CAD build for the part. Positions are in the model's coordinates, mm. A direction names the side the tool comes from. Round coordinates to 2 decimals unless told otherwise and drop trailing zeros. Write each loop counter-clockwise with the first axis right and the second up, starting at its lowest first coordinate (ties: lowest second). Pieces come first, ordered by that corner, then holes. Notation, with made-up numbers: (-4.5, -24.75) -> (15.5, -24.75) arc R19 cw to (15.5, 3.25) -> close; hole circle Ø10 at (-15, 42). An arc over 180 degrees is marked (long way). Answer in a Markdown table with one row per item. Add a question column.
```python
from build123d import *

# Parameters (mm, degrees)
SKETCH1_W                 = 79
SKETCH1_H                 = 62
SKETCH1_W_2               = 69
SKETCH1_H_2               = 52
BOSS_EXTRUDE1_DEPTH       = 24.3
BOSS_EXTRUDE2_START       = -5
BOSS_EXTRUDE2_OUTLINE_W   = 79
BOSS_EXTRUDE2_OUTLINE_H   = 62
BOSS_EXTRUDE2_OUTLINE_W_2 = 74
BOSS_EXTRUDE2_OUTLINE_H_2 = 57
BOSS_EXTRUDE2_DEPTH       = 5
SKETCH3_W                 = 10
SKETCH3_H                 = 2.5
BOSS_EXTRUDE3_DEPTH       = 7.5
CUT_EXTRUDE1_DEPTH        = 63.355753544
CUT_EXTRUDE1_DEPTH_BACK   = 63.355753544
SKETCH4_R                 = 1.5
FILLET1_R                 = 15


# Read off the part's stored shape, not the designer's step: Boss-Extrude2
with BuildPart() as part:
    # Sketch1 → Boss-Extrude1 (new body)
    with BuildSketch(Plane(origin=(0, 0, 0), x_dir=(1, 0, 0), z_dir=(0, 1, 0))):
        Rectangle(SKETCH1_W, SKETCH1_H)
        Rectangle(SKETCH1_W_2, SKETCH1_H_2, mode=Mode.SUBTRACT)
    extrude(amount=BOSS_EXTRUDE1_DEPTH)

    # Boss-Extrude2 outline → Boss-Extrude2 (add)
    with BuildSketch(Plane(origin=(0, 0, 0), x_dir=(1, 0, 0), z_dir=(0, 1, 0)).offset(BOSS_EXTRUDE2_START)):
        Rectangle(BOSS_EXTRUDE2_OUTLINE_W, BOSS_EXTRUDE2_OUTLINE_H)
        Rectangle(BOSS_EXTRUDE2_OUTLINE_W_2, BOSS_EXTRUDE2_OUTLINE_H_2, mode=Mode.SUBTRACT)
    extrude(amount=BOSS_EXTRUDE2_DEPTH)

    # Sketch3 → Boss-Extrude3 (add)
    with BuildSketch(Plane.ZY.offset(39.5)):
        with Locations((-26, 23.05)):
            Rectangle(SKETCH3_W, SKETCH3_H)
        with Locations((26, 23.05)):
            Rectangle(SKETCH3_W, SKETCH3_H)
    boss_extrude3 = extrude(amount=BOSS_EXTRUDE3_DEPTH)

    # Mirror1: Boss-Extrude3 across plane
    add(boss_extrude3.mirror(Plane.ZY))

    # Sketch4 → Cut-Extrude1 (cut, two sides: drawn at the far end of the back side and taken through both)
    with BuildSketch(Plane.XZ.offset(-21.8).offset(-CUT_EXTRUDE1_DEPTH_BACK)):
        with Locations(Location((43.25, 26, 0), (0, 0, 270))):
            Circle(SKETCH4_R)
        with Locations(Location((-43.25, 26, 0), (0, 0, 90))):
            Circle(SKETCH4_R)
        with Locations(Location((-43.25, -26, 0), (0, 0, 270))):
            Circle(SKETCH4_R)
        with Locations(Location((43.25, -26, 0), (0, 0, 270))):
            Circle(SKETCH4_R)
    extrude(amount=CUT_EXTRUDE1_DEPTH + CUT_EXTRUDE1_DEPTH_BACK, mode=Mode.SUBTRACT)

    # Fillet1
    # the kernel refuses this fillet: 15 mm, written as the material it takes off along each edge
    with BuildSketch(Plane(origin=(-77, -5, 31), x_dir=(0, 1, 0), z_dir=(1, 0, 0))) as fillet1_piece_1:
        with BuildLine():
            CenterArc((FILLET1_R, -FILLET1_R), FILLET1_R, 90, 90)
            Line((0, -FILLET1_R), (-FILLET1_R * 0.02, -FILLET1_R))
            Line((-FILLET1_R * 0.02, -FILLET1_R), (-FILLET1_R * 0.02, FILLET1_R * 0.02))
            Line((-FILLET1_R * 0.02, FILLET1_R * 0.02), (FILLET1_R, FILLET1_R * 0.02))
            Line((FILLET1_R, FILLET1_R * 0.02), (FILLET1_R, 0))
        make_face()
    extrude(amount=154, mode=Mode.SUBTRACT)
    # the kernel refuses this fillet: 15 mm, written as the material it takes off along each edge
    with BuildSketch(Plane(origin=(77, -5, -31), x_dir=(0, 1, 0), z_dir=(-1, 0, 0))) as fillet1_2_piece_1:
        with BuildLine():
            CenterArc((FILLET1_R, -FILLET1_R), FILLET1_R, 90, 90)
            Line((0, -FILLET1_R), (-FILLET1_R * 0.02, -FILLET1_R))
            Line((-FILLET1_R * 0.02, -FILLET1_R), (-FILLET1_R * 0.02, FILLET1_R * 0.02))
            Line((-FILLET1_R * 0.02, FILLET1_R * 0.02), (FILLET1_R, FILLET1_R * 0.02))
            Line((FILLET1_R, FILLET1_R * 0.02), (FILLET1_R, 0))
        make_face()
    extrude(amount=154, mode=Mode.SUBTRACT)


solid = part.part
```
Item 1: Pin check, flat tips, straight feed: pin 1 (1.5 mm diameter, centred on y = 10.5, z = -17, fed in from -X); pin 2 (2.5 mm diameter, centred on x = -43.25, z = -26, fed in from +Y); pin 3 (8 mm diameter, centred on x = -42.5, z = 25.5, fed in from -Y); pin 4 (1.5 mm diameter, centred on y = 3.5, z = -16, fed in from +X). Stop position of each tip, or through.
Item 2: Saw through at B-B on x = 43.25. Give the cut face in (y, z), then the cut area to 3 significant figures.
Item 3: Saw through at C-C on z = -8.5. Give the cut face in (x, y), then the cut area to 3 significant figures.
Item 4: Saw through at D-D on y = 9. Give the cut face in (x, z).
Item 5: Drill centre lines: probe 1 along X at (y, z) = (4.75, 23); probe 2 along Z at (x, y) = (31, 14); probe 3 along X at (y, z) = (-1, 19). Where is each one in solid material? Low to high.
Item 6: Saw through at A-A on x = -1.5. Give the cut face in (y, z), then the cut area to 3 significant figures.
Item 7: Tool access for faces 4 (the flat face through (43, 23, -21)), 5 (the flat face through (-37, -3, 0)), 6 (the flat face through (45, 21.8, -26)), 7 (the flat face through (-34.5, 12, 0)): list every direction of +Z, -Z, +X, -X, +Y, -Y with a clear straight run to the whole face (end or side of a thin tool).
Item 8: Two-plate mould, pull along Z, no slides. Class faces 1 (the flat face through (-0.2, 0, -26.3)), 2 (the cylindrical face through (0.55, 6.28, -30.53)), 3 (the flat face through (0, 12, 26)): +Z half, -Z half, draft (parallel to the pull), parting line (faces both ways), or undercut.
Recorded:
| question | item | result |
|---|---|---|
| 1 | pin 1 | x = -39.5 |
| 1 | pin 2 | through |
| 1 | pin 3 | y = -3.34 |
| 1 | pin 4 | x = 39.5 |
| 2 | outline | (21.8, -31) -> (24.3, -31) -> (24.3, -27.5) -> (21.8, -27.5) -> close; (21.8, -24.5) -> (24.3, -24.5) -> (24.3, -21) -> (21.8, -21) -> close; (21.8, 21) -> (24.3, 21) -> (24.3, 24.5) -> (21.8, 24.5) -> close; (21.8, 27.5) -> (24.3, 27.5) -> (24.3, 31) -> (21.8, 31) -> close |
| 2 | area | 35.0 mm2 |
| 3 | outline | (-39.5, -5) -> (-37, -5) -> (-37, 0) -> (-34.5, 0) -> (-34.5, 24.3) -> (-39.5, 24.3) -> close; (34.5, 0) -> (37, 0) -> (37, -5) -> (39.5, -5) -> (39.5, 24.3) -> (34.5, 24.3) -> close |
| 3 | area | 268 mm2 |
| 4 | outline | (-39.5, -30.97) -> (39.5, -30.97) -> (39.5, 30.97) -> (-39.5, 30.97) -> close; hole (-34.5, -26) -> (34.5, -26) -> (34.5, 26) -> (-34.5, 26) -> close |
| 5 | probe 1 | -39.5 to -34.5, 34.5 to 39.5 |
| 5 | probe 2 | -31 to -26, 26 to 31 |
| 5 | probe 3 | -39.5 to -37, 37 to 39.5 |
| 6 | outline | (0, -27.18) arc R15 ccw to (10, -31) -> (24.3, -31) -> (24.3, -26) -> (0, -26) -> close; (0, 26) -> (24.3, 26) -> (24.3, 31) -> (10, 31) arc R15 ccw to (0, 27.18) -> close |
| 6 | area | 219 mm2 |
| 7 | face 4 | +X, +Y, -Y |
| 7 | face 5 | +Z, -Z, -Y |
| 7 | face 6 | +Z, -Z, +X, -Y |
| 7 | face 7 | +Y, -Y |
| 8 | face 1 | draft |
| 8 | face 2 | -Z half |
| 8 | face 3 | undercut |
